Source: CAD feature listing. Evaluate the final solid. Frame: model axes, mm. A direction names the side the tool comes from. Round coordinates to 2 decimals unless told otherwise and drop trailing zeros. Order: outer loops, then holes, each group sorted by start corner. A loop starts at its lowest first (then second) coordinate and runs counter-clockwise, first axis right, second up. Notation, with made-up numbers: (-26, 25.5) -> (28, 25.5) arc R32 cw to (28, 64.5) -> close; hole circle Ø8 at (-39.75, 27). An arc over 180 degrees is marked (long way). One line per item, written item: value. Start each with the question number.
1) Section B-B (z = 0). Return the cut outline in (x, y).
2) Pin query (flat end, axial travel): P1, Ø2, axis at x = -2.5, z = 35, coming from the +Y side; P2, Ø4, axis at y = 4, z = 6, coming from the -X side; P3, Ø0.7, axis at x = 26.5, z = 1, coming from the +Y side. Return the tip coordinate at first contact, or that it passes through.
3) Section C-C (x = -11). Return the cut outline in (y, z).
4) Section D-D (z = -20). Return the cut outline in (x, y), and give its area (3 significant figures).
5) Reachability of faces 1 (the face through (-4.25, 3, -38)), 2 (the face through (4.25, 3, -38)), 3 (the face through (27, 9, 0)) from +Z, -Z, +X, -X, +Y, -Y: full face, straight path, thin tool, end or side. Return the list, or none.
6) Section A-A (y = 7.5). Return the cut outline in (x, z).
7) Ray query, L1, parallel to X at y = 13, z = 0; L2, parallel to Y at x = 0, z = -22.5; L3, parallel to X at y = 3.25, z = -31. Return the intervals inside material, ascending.
```python
from build123d import *

# Parameters (mm, degrees)
SKETCH1_R           = 31.06
BOSS_EXTRUDE1_DEPTH = 16
SKETCH2_R           = 28.06
CUT_EXTRUDE1_DEPTH  = 14
BOSS_EXTRUDE2_DEPTH = 7
CUT_EXTRUDE2_DEPTH  = 47.748766829
SKETCH5_W           = 2
SKETCH5_H           = 12.000963959
CUT_EXTRUDE3_DEPTH  = 47.748766998
BOSS_EXTRUDE3_DEPTH = 18
BOSS_EXTRUDE4_DEPTH = 18
CUT_EXTRUDE4_DEPTH  = 9.75


with BuildPart() as part:
    # Sketch1 → Boss-Extrude1 (new body)
    with BuildSketch(Plane(origin=(0, 0, 0), x_dir=(1, 0, 0), z_dir=(0, 1, 0))):
        with Locations(Location((0, 0, 0), (0, 0, 270))):
            Circle(SKETCH1_R)
    extrude(amount=BOSS_EXTRUDE1_DEPTH)

    # Sketch2 → Cut-Extrude1 (cut)
    with BuildSketch(Plane(origin=(0, 16, 0), x_dir=(1, 0, 0), z_dir=(0, 1, 0))):
        with Locations(Location((0, 0, 0), (0, 0, 270))):
            Circle(SKETCH2_R)
    extrude(amount=-CUT_EXTRUDE1_DEPTH, mode=Mode.SUBTRACT)

    # Sketch3 → Boss-Extrude2 (add)
    with BuildSketch(Plane(origin=(0, 2, 0), x_dir=(1, 0, 0), z_dir=(0, 1, 0))):
        with BuildLine():
            ThreePointArc((-27.961594797, -2.347938759), (-25.71, 0), (-27.961594797, 2.347938759))
            ThreePointArc((-27.961594797, 2.347938759), (-28.06, 0), (-27.961594797, -2.347938759))
        make_face()
        with BuildLine():
            ThreePointArc((27.961594797, 2.347938759), (25.71, 0), (27.961594797, -2.347938759))
            ThreePointArc((27.961594797, -2.347938759), (28.06, 0), (27.961594797, 2.347938759))
        make_face()
    extrude(amount=BOSS_EXTRUDE2_DEPTH)

    # Sketch4 → Cut-Extrude2 (cut, through all)
    with BuildSketch(Plane.XY):
        with BuildLine():
            Line((2.75, 6.25), (2.75, 16))
            Line((2.75, 16), (-2.75, 16))
            Line((-2.75, 16), (-2.75, 6.25))
            ThreePointArc((-2.75, 6.25), (-1.944543648, 4.305456352), (0, 3.5))
            ThreePointArc((0, 3.5), (1.944543648, 4.305456352), (2.75, 6.25))
        make_face()
    extrude(amount=-CUT_EXTRUDE2_DEPTH, mode=Mode.SUBTRACT)

    # Sketch5 → Cut-Extrude3 (cut, through all)
    with BuildSketch(Plane.XY):
        with Locations((0.098176677, 9.999518021)):
            Rectangle(SKETCH5_W, SKETCH5_H)
    extrude(amount=CUT_EXTRUDE3_DEPTH, mode=Mode.SUBTRACT)

    # Sketch6 → Boss-Extrude3 (add)
    with BuildSketch(Plane.XY.offset(-28.06)):
        with BuildLine():
            Line((-4.25, 0), (4.25, 0))
            Line((4.25, 0), (4.25, 6.25))
            Line((4.25, 6.25), (2.75, 6.25))
            ThreePointArc((2.75, 6.25), (0, 3.5), (-2.75, 6.25))
            Line((-2.75, 6.25), (-4.25, 6.25))
            Line((-4.25, 6.25), (-4.25, 0))
        make_face()
    extrude(amount=-BOSS_EXTRUDE3_DEPTH)

    # Sketch7 → Boss-Extrude4 (add)
    with BuildSketch(Plane(origin=(0, 0, 28.06), x_dir=(-1, 0, 0), z_dir=(0, 0, -1))):
        with BuildLine():
            Line((4.25, 6.25), (1.5, 6.25))
            ThreePointArc((1.5, 6.25), (0, 4.75), (-1.5, 6.25))
            Line((-1.5, 6.25), (-4.25, 6.25))
            Line((-4.25, 6.25), (-4.25, 0))
            Line((-4.25, 0), (4.25, 0))
            Line((4.25, 0), (4.25, 6.25))
        make_face()
    extrude(amount=-BOSS_EXTRUDE4_DEPTH)

    # Sketch8 → Cut-Extrude4 (cut)
    with BuildSketch(Plane(origin=(0, 16, 0), x_dir=(1, 0, 0), z_dir=(0, 1, 0))):
        with BuildLine():
            Line((2.75, 27.924918979), (2.75, 30.938020299))
            Line((2.75, 30.938020299), (6.357775263, 27.330245036))
            ThreePointArc((6.357775263, 27.330245036), (4.563584319, 27.686409991), (2.75, 27.924918979))
        make_face()
        with BuildLine():
            Line((-2.75, 27.924918979), (-2.75, 30.938020299))
            Line((-2.75, 30.938020299), (-6.357775263, 27.330245036))
            ThreePointArc((-6.357775263, 27.330245036), (-4.563584319, 27.686409991), (-2.75, 27.924918979))
        make_face()
    extrude(amount=-CUT_EXTRUDE4_DEPTH, mode=Mode.SUBTRACT)


solid = part.part
```
Findings:
1. outline: (-31.06, 0) -> (31.06, 0) -> (31.06, 16) -> (28.06, 16) -> (28.06, 9) -> (25.71, 9) -> (25.71, 2) -> (-25.71, 2) -> (-25.71, 9) -> (-28.06, 9) -> (-28.06, 16) -> (-31.06, 16) -> close
2. P1: y = 6.25
2. P2: x = -30.8
2. P3: y = 9
3. outline: (0, -29.05) -> (16, -29.05) -> (16, -25.81) -> (2, -25.81) -> (2, 25.81) -> (16, 25.81) -> (16, 29.05) -> (0, 29.05) -> close
4. outline: (-23.76, 0) -> (23.76, 0) -> (23.76, 16) -> (19.68, 16) -> (19.68, 2) -> (-19.68, 2) -> (-19.68, 16) -> (-23.76, 16) -> close
4. area: 209 mm2
5. face 1: -Z, -X, +Y, -Y
5. face 2: -Z, +X, +Y, -Y
5. face 3: +Y
6. outline: (-27.96, -2.35) arc R2.35 ccw to (-27.96, 2.35) arc R28.06 cw to (-0.9, 28.05) -> (-0.9, 31.05) arc R31.06 ccw to (-2.75, -30.94) -> (-6.36, -27.33) arc R28.06 cw to start; (1.1, 28.04) arc R28.06 cw to (27.96, 2.35) arc R2.35 ccw to (27.96, -2.35) arc R28.06 cw to (6.36, -27.33) -> (2.75, -30.94) arc R31.06 ccw to (1.1, 31.04) -> close
7. L1: -31.06 to -28.06, 28.06 to 31.06
7. L2: 0 to 2
7. L3: -4.25 to 4.25
